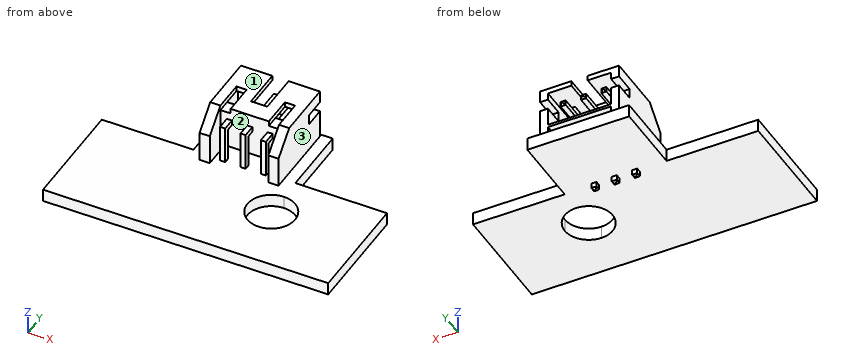
```python
from build123d import *

# Parameters (mm, degrees)
CROQUIS1_W          = 10
CROQUIS1_H          = 7
EXTRUIR1_DEPTH      = 1.25
CROQUIS2_W          = 7.75
CROQUIS2_H          = 7.75
EXTRUIR2_DEPTH      = 5
CROQUIS3_W          = 6.199548142
CROQUIS3_H          = 3.5
EXTRUIR3_DEPTH      = 4.5
CROQUIS4_W          = 5.75
CROQUIS4_H          = 2
EXTRUIR4_DEPTH      = 5
CHAFL_N1_SIZE       = 2
CROQUIS5_W          = 6.199548142
CROQUIS5_H          = 0.75
EXTRUIR5_DEPTH      = 5.75
CROQUIS6_W          = 1
CROQUIS6_H          = 3
CROQUIS6_W_2        = 0.8
CROQUIS6_H_2        = 4
EXTRUIR6_DEPTH      = 0.5
EXTRUIR7_REACH      = 24.69
CROQUIS7_W          = 1
CROQUIS7_H          = 2
EXTRUIR8_DEPTH      = 4
EXTRUIR8_DEPTH_BACK = 2.5
CROQUIS8_W          = 0.5
CROQUIS8_H          = 0.5
CHAFL_N2_SIZE       = 0.25
CROQUIS9_W          = 0.5
CROQUIS9_H          = 0.5
EXTRUIR9_DEPTH      = 5.75
CHAFL_N3_SIZE       = 0.25


with BuildPart() as part:
    # Croquis1 → Extruir1 (new body)
    with BuildSketch(Plane.XY):
        with BuildLine():
            Line((-14, -5.5), (14, -5.5))
            Line((14, -5.5), (14, 5.5))
            Line((14, 5.5), (5, 5.5))
            Line((5, 5.5), (5, 3.35))
            ThreePointArc((5, 3.35), (6.661700936, 2.661700936), (7.35, 1))
            ThreePointArc((7.35, 1), (6.661700936, -0.661700936), (5, -1.35))
            Line((5, -1.35), (5, -1.5))
            Line((5, -1.5), (-5, -1.5))
            Line((-5, -1.5), (-5, 5.5))
            Line((-5, 5.5), (-14, 5.5))
            Line((-14, 5.5), (-14, -5.5))
        make_face()
        with Locations((0, 9)):
            Rectangle(CROQUIS1_W, CROQUIS1_H)
        with BuildLine():
            Line((5, 3.35), (5, 5.5))
            Line((5, 5.5), (-5, 5.5))
            Line((-5, 5.5), (-5, -1.5))
            Line((-5, -1.5), (5, -1.5))
            Line((5, -1.5), (5, -1.35))
            ThreePointArc((5, -1.35), (2.65, 1), (5, 3.35))
        make_face()
    extrude(amount=EXTRUIR1_DEPTH)

    # Croquis2 → Extruir2 (add)
    with BuildSketch(Plane.XY.offset(1.25)):
        with Locations((0, 8.375)):
            Rectangle(CROQUIS2_W, CROQUIS2_H)
    extrude(amount=EXTRUIR2_DEPTH)

    # Croquis3 → Extruir3 (cut)
    with BuildSketch(Plane(origin=(0, 12.25, 0), x_dir=(-1, 0, 0), z_dir=(0, 1, 0))):
        with Locations((0, 4)):
            Rectangle(CROQUIS3_W, CROQUIS3_H)
    extrude(amount=-EXTRUIR3_DEPTH, mode=Mode.SUBTRACT)

    # Croquis4 → Extruir4 (cut)
    with BuildSketch(Plane.XY.offset(6.25)):
        with Locations((0, 5.5)):
            Rectangle(CROQUIS4_W, CROQUIS4_H)
    extrude(amount=-EXTRUIR4_DEPTH, mode=Mode.SUBTRACT)

    # Chaflán1
    chafl_n1_edges = [part.edges().sort_by_distance(p)[0] for p in [
        (3.375, 4.5, 6.25),
        (-3.375, 4.5, 6.25),
    ]]
    chamfer(chafl_n1_edges, length=CHAFL_N1_SIZE)

    # Croquis5 → Extruir5 (cut)
    with BuildSketch(Plane(origin=(0, 12.25, 0), x_dir=(-1, 0, 0), z_dir=(0, 1, 0))):
        with Locations((0, 1.625)):
            Rectangle(CROQUIS5_W, CROQUIS5_H)
    extrude(amount=-EXTRUIR5_DEPTH, mode=Mode.SUBTRACT)

    # Croquis6 → Extruir6 (cut)
    with BuildSketch(Plane.XY.offset(6.25)):
        with Locations((-2.375, 8)):
            Rectangle(CROQUIS6_W, CROQUIS6_H)
        with Locations((0.4, 10.25)):
            Rectangle(CROQUIS6_W_2, CROQUIS6_H_2)
        with Locations((-0.4, 10.25)):
            Rectangle(CROQUIS6_W_2, CROQUIS6_H_2)
        with Locations((2.375, 8)):
            Rectangle(CROQUIS6_W, CROQUIS6_H)
    extrude(amount=-EXTRUIR6_DEPTH, mode=Mode.SUBTRACT)

    # Extruir7: up to this face of the body (flat: up to its plane)
    extruir7_end = Plane(part.part.faces().sort_by_distance((-3.875, 8.549603175, 3.650226757))[0])
    # Croquis7 → Extruir7 (cut, up to the picked face)
    with BuildSketch(Plane(origin=(3.875, 0, 0), x_dir=(0, 0, -1), z_dir=(1, 0, 0)), mode=Mode.PRIVATE) as extruir7_sk1:
        with Locations((-4.55, 11.25)):
            Rectangle(CROQUIS7_W, CROQUIS7_H)
    extruir7_tool1 = split(extrude(extruir7_sk1.sketch, amount=-EXTRUIR7_REACH, mode=Mode.PRIVATE), bisect_by=extruir7_end, keep=Keep.BOTH, mode=Mode.PRIVATE)
    add(extruir7_tool1.solids().sort_by(Axis((3.875, 11.25, 4.55), (-1, 0, 0)))[0], mode=Mode.SUBTRACT)

    # Croquis8 → Extruir8 (add, two sides: drawn at the far end of the back side and taken through both)
    with BuildSketch(Plane(origin=(0, 7.75, 0), x_dir=(-1, 0, 0), z_dir=(0, 1, 0)).offset(-EXTRUIR8_DEPTH_BACK)):
        with Locations((0, 4.75)):
            Rectangle(CROQUIS8_W, CROQUIS8_H)
        with Locations((2, 4.75)):
            Rectangle(CROQUIS8_W, CROQUIS8_H)
        with Locations((-2, 4.75)):
            Rectangle(CROQUIS8_W, CROQUIS8_H)
    extrude(amount=EXTRUIR8_DEPTH + EXTRUIR8_DEPTH_BACK)

    # Chaflán2
    chafl_n2_edges = [part.edges().sort_by_distance(p)[0] for p in [
        (0.25, 11.75, 4.75),
        (0, 11.75, 4.5),
        (-0.25, 11.75, 4.75),
        (0, 11.75, 5),
        (-1.75, 11.75, 4.75),
        (-2, 11.75, 4.5),
        (-2.25, 11.75, 4.75),
        (-2, 11.75, 5),
        (1.75, 11.75, 4.75),
        (2, 11.75, 5),
        (2.25, 11.75, 4.75),
        (2, 11.75, 4.5),
    ]]
    chamfer(chafl_n2_edges, length=CHAFL_N2_SIZE - 0.0001)  # a hair under: the kernel refuses the full size

    # Croquis9 → Extruir9 (add)
    with BuildSketch(Plane.XY.offset(5)):
        with Locations((-2, 5.5)):
            Rectangle(CROQUIS9_W, CROQUIS9_H)
        with Locations((0, 5.5)):
            Rectangle(CROQUIS9_W, CROQUIS9_H)
        with Locations((2, 5.5)):
            Rectangle(CROQUIS9_W, CROQUIS9_H)
    extrude(amount=-EXTRUIR9_DEPTH)

    # Chaflán3
    chafl_n3_edges = [part.edges().sort_by_distance(p)[0] for p in [
        (-2, 5.25, -0.75),
        (-2, 5.75, -0.75),
        (-1.75, 5.5, -0.75),
        (-2.25, 5.5, -0.75),
        (0, 5.75, -0.75),
        (0, 5.25, -0.75),
        (-0.25, 5.5, -0.75),
        (0.25, 5.5, -0.75),
        (2, 5.75, -0.75),
        (2, 5.25, -0.75),
        (1.75, 5.5, -0.75),
        (2.25, 5.5, -0.75),
    ]]
    chamfer(chafl_n3_edges, length=CHAFL_N3_SIZE - 0.0001)  # a hair under: the kernel refuses the full size


solid = part.part
```
CAD build for the part. Positions are in the model's coordinates, mm. Face numbers are marked on the shaded views. Coordinates: 2 decimals unless noted, no trailing zeros. Write each loop counter-clockwise with the first axis right and the second up, starting at its lowest first coordinate (ties: lowest second). Pieces come first, ordered by that corner, then holes. Notation, with made-up numbers: (38.25, 63) -> (63.25, 63) arc R25 cw to (63.25, 77) -> close; hole circle Ø9 at (77.25, 85.5). An arc over 180 degrees is marked (long way). Use CSV: the item, a comma, the result in double quotes. Start each with the question number.
Item 1: Band-saw the part on B-B, the plane y = 2.5. Write the cut outline in (x, z), plus the area to 3 significant figures.
Item 2: Band-saw the part on A-A, the plane z = 0.75. Write the cut outline in (x, y).
Item 3: Drop flat-ended pins along their axis: P1, Ø1.8, axis at y = 9, z = 3.5, coming from the -X side (3 decimals); P2, Ø1.5, axis at x = -4, y = 4.5, coming from the +Z side; P3, Ø1, axis at x = -4, z = 2, coming from the -Y side. Give the stop position or say it passes through.
Item 4: Two-plate mould, pull along X, no slides. Class the marked faces 1, 2 and 3: +X half, -X half, draft (parallel to the pull), parting line (faces both ways), or undercut.
Item 5: Wall check: probe 1 along X at (y, z) = (9.75, 3.5) (3 decimals); probe 2 along Z at (x, y) = (-7.25, 1.5); probe 3 along Y at (x, z) = (1.5, 3.5). Give the ranges that are in metal, low to high.
Item 6: Band-saw the part on C-C, the plane x = -10. Write the cut outline in (y, z), plus the area to 4 significant figures.
Response values:
1,outline,"(-14, 0) -> (3.19, 0) -> (3.19, 1.25) -> (-14, 1.25) -> close; (6.81, 0) -> (14, 0) -> (14, 1.25) -> (6.81, 1.25) -> close"
1,area,"30.5 mm2"
2,outline,"(-14, -5.5) -> (14, -5.5) -> (14, 5.5) -> (5, 5.5) -> (5, 12.5) -> (-5, 12.5) -> (-5, 5.5) -> (-14, 5.5) -> close; hole circle Ø4.7 at (5, 1)"
3,P1,"stops at x = -3.875"
3,P2,"stops at z = 4.99"
3,P3,"stops at y = 4.5"
4,face 1,"draft"
4,face 2,"undercut"
4,face 3,"+X half"
5,probe 1,"x = -3.875 to -3.1, 3.1 to 3.875"
5,probe 2,"z = 0 to 1.25"
5,probe 3,"y = 6.5 to 7.75"
6,outline,"(-5.5, 0) -> (5.5, 0) -> (5.5, 1.25) -> (-5.5, 1.25) -> close"
6,area,"13.75 mm2"
